```python
from build123d import *

# Parameters (mm, degrees)
BOSS_EXTRUDE2_DEPTH = 9.144
SKETCH2_W           = 6.604
SKETCH2_H           = 8.128
CUT_EXTRUDE1_DEPTH  = 49.022
CUT_EXTRUDE3_DEPTH  = 39.635145062
CUT_EXTRUDE4_DEPTH  = 4.064
SKETCH7_W           = 12.7
SKETCH7_H           = 1.27
BOSS_EXTRUDE3_DEPTH = 0.762
FILLET1_R           = 0.762


with BuildPart() as part:
    # Sketch1 → Boss-Extrude2 (new body)
    with BuildSketch(Plane(origin=(0, 0, 0), x_dir=(1, 0, 0), z_dir=(0, 1, 0))):
        with BuildLine():
            Line((-24.003, -26.543), (24.003, -26.543))
            ThreePointArc((24.003, -26.543), (25.799051224, -25.799051224), (26.543, -24.003))
            Line((26.543, -24.003), (26.543, 24.003))
            ThreePointArc((26.543, 24.003), (25.799051224, 25.799051224), (24.003, 26.543))
            Line((24.003, 26.543), (-24.003, 26.543))
            ThreePointArc((-24.003, 26.543), (-25.799051224, 25.799051224), (-26.543, 24.003))
            Line((-26.543, 24.003), (-26.543, -24.003))
            ThreePointArc((-26.543, -24.003), (-25.799051224, -25.799051224), (-24.003, -26.543))
        make_face()
    extrude(amount=BOSS_EXTRUDE2_DEPTH)

    # Sketch2 → Cut-Extrude1 (cut)
    with BuildSketch(Plane.XY.offset(26.543)):
        with Locations((12.827, 0)):
            Rectangle(SKETCH2_W, SKETCH2_H)
        with Locations((-12.827, 0)):
            Rectangle(SKETCH2_W, SKETCH2_H)
    extrude(amount=-CUT_EXTRUDE1_DEPTH, mode=Mode.SUBTRACT)

    # Sketch5 → Cut-Extrude3 (cut, through all)
    with BuildSketch(Plane(origin=(0, 9.144, 0), x_dir=(1, 0, 0), z_dir=(0, 1, 0))):
        with BuildLine():
            Line((-19.939, -22.479), (19.939, -22.479))
            ThreePointArc((19.939, -22.479), (21.735051224, -21.735051224), (22.479, -19.939))
            Line((22.479, -19.939), (22.479, 19.939))
            ThreePointArc((22.479, 19.939), (21.735051224, 21.735051224), (19.939, 22.479))
            Line((19.939, 22.479), (-19.939, 22.479))
            ThreePointArc((-19.939, 22.479), (-21.735051224, 21.735051224), (-22.479, 19.939))
            Line((-22.479, 19.939), (-22.479, -19.939))
            ThreePointArc((-22.479, -19.939), (-21.735051224, -21.735051224), (-19.939, -22.479))
        make_face()
    extrude(amount=-CUT_EXTRUDE3_DEPTH, mode=Mode.SUBTRACT)

    # Sketch6 → Cut-Extrude4 (cut)
    with BuildSketch(Plane(origin=(0, 9.144, 0), x_dir=(1, 0, 0), z_dir=(0, 1, 0))):
        with BuildLine():
            Line((-21.59, -24.13), (21.59, -24.13))
            ThreePointArc((21.59, -24.13), (23.386051224, -23.386051224), (24.13, -21.59))
            Line((24.13, -21.59), (24.13, 21.59))
            ThreePointArc((24.13, 21.59), (23.386051224, 23.386051224), (21.59, 24.13))
            Line((21.59, 24.13), (-21.59, 24.13))
            ThreePointArc((-21.59, 24.13), (-23.386051224, 23.386051224), (-24.13, 21.59))
            Line((-24.13, 21.59), (-24.13, -21.59))
            ThreePointArc((-24.13, -21.59), (-23.386051224, -23.386051224), (-21.59, -24.13))
        make_face()
    extrude(amount=-CUT_EXTRUDE4_DEPTH, mode=Mode.SUBTRACT)

    # Sketch7 → Boss-Extrude3 (add)
    with BuildSketch(Plane.XY.offset(-24.13)):
        with Locations((0, 7.239)):
            Rectangle(SKETCH7_W, SKETCH7_H)
    extrude(amount=BOSS_EXTRUDE3_DEPTH)

    # Fillet1
    fillet1_edges = [part.edges().sort_by_distance(p)[0] for p in [
        (0, 6.604, -23.368),
    ]]
    fillet(fillet1_edges, radius=FILLET1_R - 0.0001)  # a hair under: the kernel refuses the full size


solid = part.part
```
Could you check a few things on this model? Use its own coordinates, in mm. A direction names the side the tool comes from. Round coordinates to 2 decimals unless told otherwise and drop trailing zeros. Loops run counter-clockwise (first coordinate to the right, second up) from the corner with the lowest first, then second, coordinate; pieces in that order, holes last. Notation, with made-up numbers: (-1, 15.25) - (51, 15.25) arc R29 ccw to (51, 39.25) - close; hole circle Ø10 at (33, 14). An arc over 180 degrees is marked (long way). Answer in a Markdown table with one row per item. Add a question column.
(1) If we section it at B-B (z = 13.5): Please give me the cut outline in (x, y), plus the area to 3 significant figures.
(2) For faces 5 (the face through (13, 4.064, 25)), 6 (the face through (24.13, 7, 0)), 7 (the face through (0, 3, -22.479)), which set-ups out of +Z, -Z, +X, -X, +Y, -Y let a thin tool reach every point of the face, with its end or its side?
(3) I need wall thicknesses on line 1 along X through (y, z) = (5, -5); line 2 along Z through (x, y) = (-15, 8). Which ranges of each line are inside material? Lowest first, please.
(4) I'm going to push flat-ended pins straight in: pin 1 (2 mm diameter, centred on x = -13.5, z = 25, fed in from -Y); pin 2 (3.5 mm diameter, centred on y = 2, z = 25, fed in from +X). Where does each tip first touch, or does it pass through?
(5) If we section it at C-C (y = 2.5): Please give me the cut outline in (x, z) (3 decimals), plus the area to 3 significant figures.
(6) If we mould it in two halves opening along X, with no side actions, what happens to faces 1 (the face through (21.72, 2.58, 21.75)), 2 (the face through (0, 5, -26.543)), 3 (the face through (26.543, 5, 0)), 4 (the face through (22.479, 3, 0))? For each: pulls with the +X half, pulls with the -X half, needs draft (parallel to the pull), parting line crosses it, or undercut.
Model answer:
| question | item | result |
|---|---|---|
| 1 | outline | (-26.54, 0) - (-22.48, 0) - (-22.48, 5.08) - (-24.13, 5.08) - (-24.13, 9.14) - (-26.54, 9.14) - close; (22.48, 0) - (26.54, 0) - (26.54, 9.14) - (24.13, 9.14) - (24.13, 5.08) - (22.48, 5.08) - close |
| 1 | area | 60.9 mm² |
| 2 | face 5 | +Z, -Y |
| 2 | face 6 | +Y |
| 2 | face 7 | +Y, -Y |
| 3 | line 1 | x = -26.54 to -22.48, 22.48 to 26.54 |
| 3 | line 2 | z = -26.54 to -24.13, 24.13 to 26.54 |
| 4 | pin 1 | stops at y = 4.06 |
| 4 | pin 2 | stops at x = 26.54 |
| 5 | outline | (-26.543, -24.003) arc R2.54 ccw to (-24.003, -26.543) - (24.003, -26.543) arc R2.54 ccw to (26.543, -24.003) - (26.543, 24.003) arc R2.54 ccw to (24.003, 26.543) - (16.129, 26.543) - (16.129, 22.479) - (19.939, 22.479) arc R2.54 cw to (22.479, 19.939) - (22.479, -19.939) arc R2.54 cw to (19.939, -22.479) - (-19.939, -22.479) arc R2.54 cw to (-22.479, -19.939) - (-22.479, 19.939) arc R2.54 cw to (-19.939, 22.479) - (-16.129, 22.479) - (-16.129, 26.543) - (-24.003, 26.543) arc R2.54 ccw to (-26.543, 24.003) - close; (-9.525, 22.479) - (9.525, 22.479) - (9.525, 26.543) - (-9.525, 26.543) - close |
| 5 | area | 743 mm² |
| 6 | face 1 | undercut |
| 6 | face 2 | needs draft |
| 6 | face 3 | pulls with the +X half |
| 6 | face 4 | undercut |
